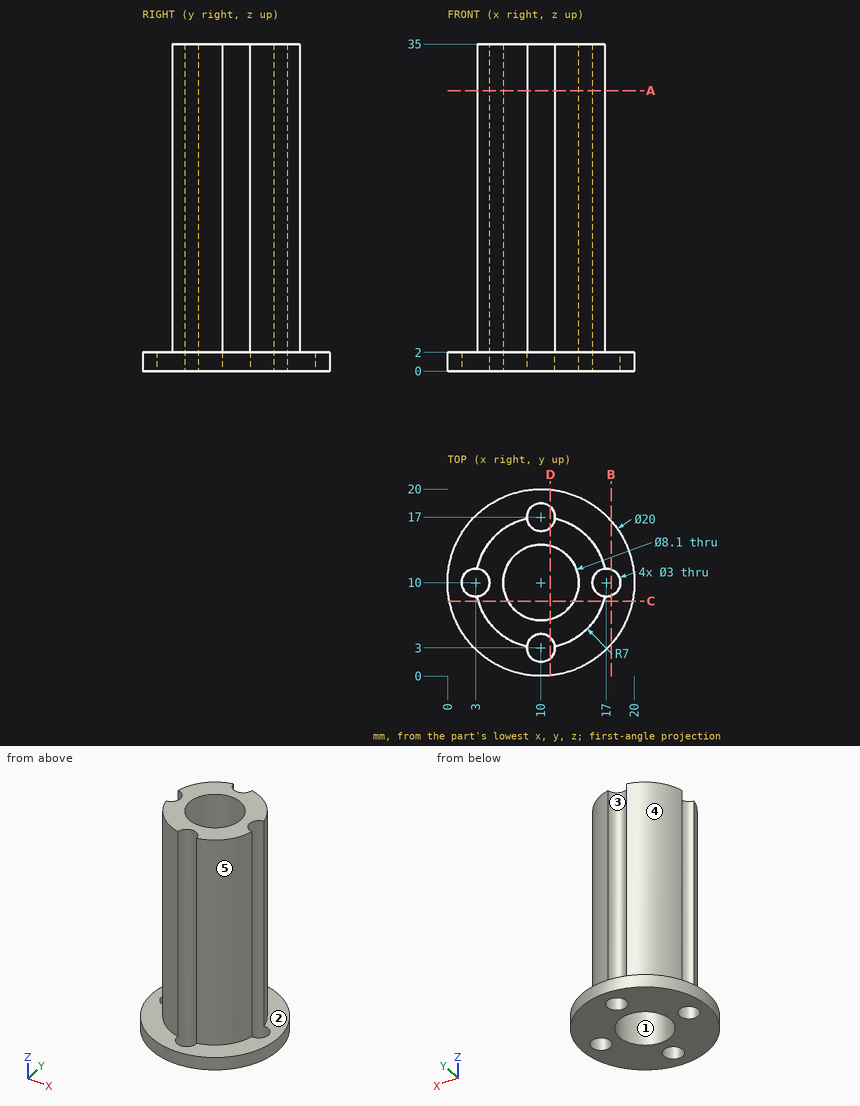
Can you work these out from the drawing? Everything is in mm from the part's minimum corner. A direction names the side the tool comes from. Give positions to 0.01 mm unless a question says otherwise; leave off trailing zeros. Write each loop counter-clockwise with the first axis right and the second up, starting at its lowest first coordinate (ties: lowest second). Pieces come first, ordered by that corner, then holes. Notation, with made-up numbers: M -21.5,89 L -1.5,89 A29 cw -1.5,125 Z; hole C 14.5,40 d5. An arc over 180 degrees is marked long. Answer in a Markdown table with one row per item. Add a question column.
Item 1: On a 3-axis mill with a long thin cutter (end or side, diameter ignored), from which of +Z, -Z, +X, -X, +Y, -Y can I reach the whole of each face in a straight line? I mean the marked faces 1 and 2. Say none if no direction works.
Item 2: Imagine slicing it at A-A, the plane z = 30. Write out the boundary of the cut face in (x, y).
Item 3: Imagine slicing it at B-B, the plane x = 17.5. Write out the boundary of the cut face in (y, z).
Item 4: Please list where these lines run through material, in increasing order: L1, parallel to Y at x = 10, z = 23; L2, parallel to X at y = 9.5, z = 8.
Item 5: Imagine slicing it at C-C, the plane y = 8. Write out the boundary of the cut face in (x, z).
Item 6: For pin 1 Ø10 at (x, z) = (15, 23.5) entering from -Y; pin 2 Ø5 at (x, y) = (3, 10) entering from -Z; pin 3 Ø1.5 at (x, z) = (12, 11) entering from +Y; pin 4 Ø2 at (y, z) = (5, 4) entering from -X, each with a flat end and sliding along its axis, tell me the tip position at first contact or that it passes through.
Item 7: Imagine slicing it at D-D, the plane x = 11. Write out the boundary of the cut face in (y, z), plus the area to 3 significant figures.
Item 8: We'd pull the mould along X, two halves only. Please class the marked faces 3, 4 and 5: released by +X, released by -X, zero draft, split by the parting line, or undercut.
Evaluation:
| question | item | result |
|---|---|---|
| 1 | face 1 | +Z, -Z |
| 1 | face 2 | +Z |
| 2 | outline | M 3.16,8.51 A7 ccw 8.51,3.16 A1.5 cw 11.49,3.16 A7 ccw 16.84,8.51 A1.5 cw 16.84,11.49 A7 ccw 11.49,16.84 A1.5 cw 8.51,16.84 A7 ccw 3.16,11.49 A1.5 cw Z; hole C 10,10 d8.1 |
| 3 | outline | M 3.39,0 L 8.59,0 L 8.59,2 L 3.39,2 Z; M 11.41,0 L 16.61,0 L 16.61,2 L 11.41,2 Z |
| 4 | L1 | y = 4.5 to 5.95, 14.05 to 15.5 |
| 4 | L2 | x = 4.41 to 5.98, 14.02 to 15.59 |
| 5 | outline | M 0.2,0 L 6.48,0 L 6.48,35 L 3.29,35 L 3.29,2 L 0.2,2 Z; M 13.52,0 L 19.8,0 L 19.8,2 L 16.71,2 L 16.71,35 L 13.52,35 Z |
| 6 | pin 1 | stops at y = 3.16 |
| 6 | pin 2 | stops at z = 0 |
| 6 | pin 3 | stops at y = 16.84 |
| 6 | pin 4 | stops at x = 4.26 |
| 7 | outline | M 0.05,0 L 1.88,0 L 1.88,2 L 0.05,2 Z; M 4.12,0 L 6.08,0 L 6.08,35 L 4.12,35 Z; M 13.92,0 L 15.88,0 L 15.88,35 L 13.92,35 Z; M 18.12,0 L 19.95,0 L 19.95,2 L 18.12,2 Z |
| 7 | area | 144 mm² |
| 8 | face 3 | undercut |
| 8 | face 4 | released by -X |
| 8 | face 5 | released by +X |
